Build history of the part. All positions in model axes, mm. Face numbers are marked on the shaded views. A direction names the side the tool comes from. Round coordinates to 2 decimals unless told otherwise and drop trailing zeros. Order: outer loops, then holes, each group sorted by start corner. A loop starts at its lowest first (then second) coordinate and runs counter-clockwise, first axis right, second up. Notation, with made-up numbers: (48.5, 34) -> (81.5, 34) arc R25 ccw to (81.5, 55) -> close; hole circle Ø2 at (-34.5, 32.25). An arc over 180 degrees is marked (long way). Write item = value, one per line.
from build123d import *

# Parameters (mm, degrees)
SKETCH1_W               = 152.4
SKETCH1_H               = 25.4
BOSS_EXTRUDE1_DEPTH     = 5.08
BOSS_EXTRUDE2_DEPTH     = 5.08
SKETCH5_W               = 162.56
SKETCH5_H               = 60.96
BOSS_EXTRUDE3_DEPTH     = 5.08
CUT_EXTRUDE2_DEPTH      = 163.56
SKETCH7_W               = 63.5
SKETCH7_H               = 38.1
BOSS_EXTRUDE4_DEPTH     = 5.08
BOSS_EXTRUDE5_DEPTH     = 6.35
CUT_EXTRUDE3_REACH      = 97.25
SKETCH9_W               = 44.45
SKETCH9_H               = 39.033619981
SKETCH10_R              = 8.2696685
CUT_EXTRUDE4_DEPTH      = 2.54
CUT_EXTRUDE4_DEPTH_BACK = 112.76


with BuildPart() as part:
    # Sketch1 → Boss-Extrude1 (new body)
    with BuildSketch(Plane(origin=(0, 0, 0), x_dir=(1, 0, 0), z_dir=(0, 1, 0))):
        Rectangle(SKETCH1_W, SKETCH1_H)
    extrude(amount=BOSS_EXTRUDE1_DEPTH)

    # Sketch4 → Boss-Extrude2 (add)
    with BuildSketch(Plane(origin=(76.2, 0, 0), x_dir=(0, 0, -1), z_dir=(1, 0, 0))):
        Polygon((-12.7, 0), (-12.7, 5.08), (-12.7, 60.96), (12.7, 60.96), (12.7, 5.08), (12.7, 0), align=None)
    boss_extrude2 = extrude(amount=BOSS_EXTRUDE2_DEPTH)

    # Mirror1: Boss-Extrude2 across plane
    add(boss_extrude2.mirror(Plane(origin=(0, 0, 0), x_dir=(0, 0, 1), z_dir=(1, 0, 0))))

    # Sketch5 → Boss-Extrude3 (add)
    with BuildSketch(Plane(origin=(0, 0, -12.7), x_dir=(-1, 0, 0), z_dir=(0, 0, -1))):
        with Locations((0, 30.48)):
            Rectangle(SKETCH5_W, SKETCH5_H)
    extrude(amount=BOSS_EXTRUDE3_DEPTH)

    # Sketch6 → Cut-Extrude2 (cut, through all)
    with BuildSketch(Plane(origin=(81.28, 0, 0), x_dir=(0, 0, -1), z_dir=(1, 0, 0))):
        Polygon((-12.7, 0), (12.7, 6.35), (-12.7, 6.35), align=None)
    extrude(amount=-CUT_EXTRUDE2_DEPTH, mode=Mode.SUBTRACT)

    # Sketch7 → Boss-Extrude4 (add)
    with BuildSketch(Plane(origin=(0, 0, -17.78), x_dir=(-1, 0, 0), z_dir=(0, 0, -1))):
        with Locations((0, 69.85)):
            Rectangle(SKETCH7_W, SKETCH7_H)
    extrude(amount=BOSS_EXTRUDE4_DEPTH)

    # Sketch8 → Boss-Extrude5 (add)
    with BuildSketch(Plane(origin=(0, 88.9, 0), x_dir=(1, 0, 0), z_dir=(0, 1, 0))):
        Polygon((-31.75, 22.86), (-31.75, 124.46), (31.75, 124.46), (31.75, 22.86), (31.75, 17.78), (31.75, -20.32), (-31.75, -20.32), (-31.75, 17.78), align=None)
    extrude(amount=BOSS_EXTRUDE5_DEPTH)

    # Sketch9 → Cut-Extrude3 (cut, up to next)
    with BuildSketch(Plane(origin=(0, 95.25, 0), x_dir=(1, 0, 0), z_dir=(0, 1, 0)), mode=Mode.PRIVATE) as cut_extrude3_sk1:
        with Locations((0, -21.646832164)):
            Rectangle(SKETCH9_W, SKETCH9_H)
    cut_extrude3_tool1 = extrude(cut_extrude3_sk1.sketch, amount=-CUT_EXTRUDE3_REACH, mode=Mode.PRIVATE) & part.part
    add(cut_extrude3_tool1.solids().sort_by_distance((0, 95.25, 21.646832))[0], mode=Mode.SUBTRACT)

    # Sketch10 → Cut-Extrude4 (cut, two sides)
    with BuildSketch(Plane.XY.offset(-12.7)) as cut_extrude4_sk:
        with Locations((-13.081, 12.7)):
            Circle(SKETCH10_R)
        with Locations((13.081, 12.7)):
            Circle(SKETCH10_R)
        with Locations((37.338, 12.7)):
            Circle(SKETCH10_R)
        with Locations((63.5, 12.7)):
            Circle(SKETCH10_R)
        with Locations((-63.5, 12.7)):
            Circle(SKETCH10_R)
        with Locations((-37.338, 12.7)):
            Circle(SKETCH10_R)
    extrude(amount=CUT_EXTRUDE4_DEPTH, mode=Mode.SUBTRACT)
    extrude(cut_extrude4_sk.sketch, amount=-CUT_EXTRUDE4_DEPTH_BACK, mode=Mode.SUBTRACT)


solid = part.part
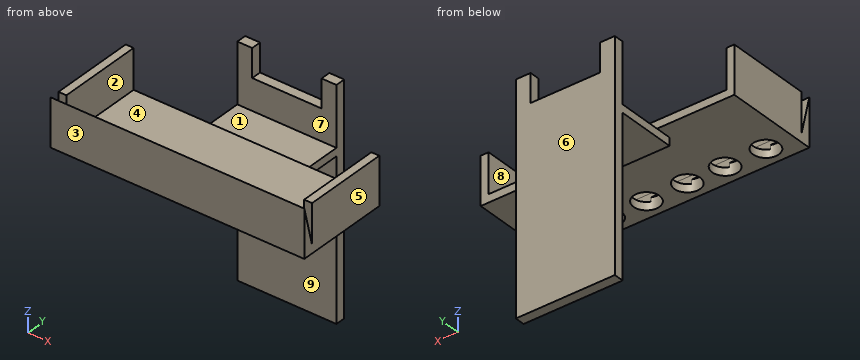
Q1. Probe probe 1 along X at (y, z) = (55, -4); probe 2 along Y at (x, z) = (2, -33); probe 3 along Y at (x, z) = (63.5, -13.75). List the from-to ranges inside material, lowest first.
Check values:
probe_1 = -81.28 to -76.2, 76.2 to 81.28
probe_2 = 88.9 to 95.25
probe_3 = 0 to 4.43, 20.97 to 60.96
Q2. Cut at D-D, the plane y = 59. List the corners of the cut face in (x, z), and give its area (3 significant figures).
Check values:
outline = (-81.28, -17.78) -> (-31.75, -17.78) -> (-31.75, -22.86) -> (31.75, -22.86) -> (31.75, -17.78) -> (81.28, -17.78) -> (81.28, 12.7) -> (76.2, 12.7) -> (76.2, -12.7) -> (-76.2, -12.7) -> (-76.2, 12.7) -> (-81.28, 12.7) -> close
area = 1,410 mm²
Q3. Mould opens along Y. For the marked faces 1, 2, 3 and 4 say: released by +Y, released by -Y, zero draft, split by the parting line, or undercut.
Check values:
face_1 = undercut
face_2 = zero draft
face_3 = released by -Y
face_4 = undercut
Q4. Cut at C-C, the plane x = 63.5. List the corners of the cut face in (y, z).
Check values:
outline = (0, -17.78) -> (4.43, -17.78) -> (4.43, -10.16) -> (5.08, -10.16) -> (5.08, -7.62) -> (0, 12.7) -> close; (20.97, -17.78) -> (60.96, -17.78) -> (60.96, -12.7) -> (20.97, -12.7) -> close
Q5. Cut at B-B, the plane z = 5.5. List the corners of the cut face in (x, y) (3 decimals), and give its area (3 significant figures).
Check values:
outline = (-81.28, 0) -> (81.28, 0) -> (81.28, 1.8) -> (-81.28, 1.8) -> close; (-81.28, 6.35) -> (-76.2, 6.35) -> (-76.2, 60.96) -> (-81.28, 60.96) -> close; (-31.75, 88.9) -> (-22.225, 88.9) -> (-22.225, 95.25) -> (-31.75, 95.25) -> close; (22.225, 88.9) -> (31.75, 88.9) -> (31.75, 95.25) -> (22.225, 95.25) -> close; (76.2, 6.35) -> (81.28, 6.35) -> (81.28, 60.96) -> (76.2, 60.96) -> close
area = 968 mm²
Q6. Flat gauge pins, fed straight in: pin 1 (4 mm diameter, centred on x = -78.5, y = 21, fed in from +Z); pin 2 (11.5 mm diameter, centred on x = -13.5, y = 62, fed in from -Z); pin 3 (3 mm diameter, centred on y = 91.5, z = 11.5, fed in from +X). Where does each tip first touch, or does it go through?
Check values:
pin_1 = 12.7
pin_2 = -22.86
pin_3 = 31.75
Q7. Which spindle directions (+Z, -Z, +X, -X, +Y, -Y) get a long thin tool onto all of the face, cutting with end or side? Do the marked faces 5, 6, 7, 8 and 9. Say none if no direction does.
Check values:
face_5 = +Z, -Z, +X, +Y, -Y
face_6 = +Z, -Z, +X, -X, +Y
face_7 = +Z, +X, -X
face_8 = +Z, +Y
face_9 = -Z, +X, -X, -Y
Q8. Cut at A-A, the plane y = 12.7. Give the number of separate pieces and of enclosed holes in the cut face, and give its area (3 significant figures).
Check values:
separate_pieces = 7
enclosed_holes = 0
area = 580 mm²
